```python
from build123d import *

# Parameters (mm, degrees)
F1_DEPTH = 304.8
F3_D     = 26.9875
F5_D     = 26.9875
F6_R     = 9.525


with BuildPart() as f1:
    # F0 (on Front) → F1 (new body)
    with BuildSketch(Plane.XZ):
        Polygon((12.7, 101.6), (0, 101.6), (0, 0), (101.6, 0), (101.6, 12.7), (12.7, 12.7), align=None)
    extrude(amount=F1_DEPTH)

    # F3 (through all)
    with Locations(Plane.YZ.offset(12.7)):
        with Locations((-266.7, 57.15), (-190.5, 57.15), (-114.3, 57.15), (-38.1, 57.15)):
            Hole(F3_D / 2)

    # F5 (through all)
    with Locations(Plane.XY.offset(12.7)):
        with Locations((57.15, -38.1), (57.15, -114.3), (57.15, -190.5), (57.15, -266.7)):
            Hole(F5_D / 2)

    # F6
    f6_edges = [f1.edges().sort_by_distance(p)[0] for p in [
        (12.7, -152.4, 101.6),
        (12.7, -152.4, 12.7),
        (101.6, -152.4, 12.7),
    ]]
    fillet(f6_edges, radius=F6_R)


solid = f1.part
```
For this review, take the finished solid that the model builds, in its own axes (mm). A direction names the side the tool comes from. Give positions to 0.01 mm unless a question says otherwise; leave off trailing zeros. Write each loop counter-clockwise with the first axis right and the second up, starting at its lowest first coordinate (ties: lowest second). Pieces come first, ordered by that corner, then holes. Notation, with made-up numbers: M 44,-3 L 85,-3 A26 cw 85,35 Z; hole C 40,6 d5. An arc over 180 degrees is marked long. Answer as CSV lines item,"result".
1. Draft analysis for pull direction X (two halves, no side actions). For faces 3 (the cylindrical face through (60.08, -279.87, 6.26)), 4 (the cylindrical face through (15.42, -154.53, 15.56)), 5 (the flat face through (28, -304.8, 10)), 6 (the cylindrical face through (58.91, -177.12, 6.26)), state which applies: +X half, -X half, draft (parallel to the pull), parting line (faces both ways), or undercut.
Findings:
face 3,"undercut"
face 4,"+X half"
face 5,"draft"
face 6,"undercut"
2. Consider section D-D, the plane y = -219. Write out the cut boundary in (x, z) (3 decimals).
Findings:
outline,"M 0,0 L 101.6,0 L 101.6,3.175 A9.525 ccw 92.075,12.7 L 22.225,12.7 A9.525 cw 12.7,22.225 L 12.7,92.075 A9.525 ccw 3.175,101.6 L 0,101.6 Z"
3. For faces 1 (the cylindrical face through (6.26, -279.57, 61.2)), 2 (the flat face through (58, -150, 12.7)), list the 3-axis set-ups (+Z, -Z, +X, -X, +Y, -Y) from which the entire face can be reached by the end or side of a thin tool; tool diameter is ignored.
Findings:
face 1,"+X, -X"
face 2,"+Z, +X, +Y, -Y"
4. Consider section C-C, the plane x = 57.15. Write out the cut boundary in (y, z), then the cut area to 3 significant figures.
Findings:
outline,"M -304.8,0 L -280.19,0 L -280.19,12.7 L -304.8,12.7 Z; M -253.21,0 L -203.99,0 L -203.99,12.7 L -253.21,12.7 Z; M -177.01,0 L -127.79,0 L -127.79,12.7 L -177.01,12.7 Z; M -100.81,0 L -51.59,0 L -51.59,12.7 L -100.81,12.7 Z; M -24.61,0 L 0,0 L 0,12.7 L -24.61,12.7 Z"
area,"2,500 mm2"
5. Consider section A-A, the plane z = 57.15. Write out the cut boundary in (x, y), then the cut area to 3 significant figures.
Findings:
outline,"M 0,-304.8 L 12.7,-304.8 L 12.7,-280.19 L 0,-280.19 Z; M 0,-253.21 L 12.7,-253.21 L 12.7,-203.99 L 0,-203.99 Z; M 0,-177.01 L 12.7,-177.01 L 12.7,-127.79 L 0,-127.79 Z; M 0,-100.81 L 12.7,-100.81 L 12.7,-51.59 L 0,-51.59 Z; M 0,-24.61 L 12.7,-24.61 L 12.7,0 L 0,0 Z"
area,"2,500 mm2"
6. Wall thickness on line 1 (Y direction, x = 3, z = 57); line 2 (X direction, y = -288, z = 79.5): over which ranges is each line inside the solid? List them lowest first.
Findings:
line 1,"y = -304.8 to -280.19, -253.21 to -203.99, -177.01 to -127.79, -100.81 to -51.59, -24.61 to 0"
line 2,"x = 0 to 12.7"
7. Consider section B-B, the plane y = -38.1. Write out the cut boundary in (x, z) (3 decimals).
Findings:
outline,"M 0,0 L 43.656,0 L 43.656,12.7 L 22.225,12.7 A9.525 cw 12.7,22.225 L 12.7,43.656 L 0,43.656 Z; M 0,70.644 L 12.7,70.644 L 12.7,92.075 A9.525 ccw 3.175,101.6 L 0,101.6 Z; M 70.644,0 L 101.6,0 L 101.6,3.175 A9.525 ccw 92.075,12.7 L 70.644,12.7 Z"
8. For pin 1 (5 mm diameter, centred on x = 58, y = -235.5, fed in from -Z); pin 2 (21 mm diameter, centred on y = -79, z = 67, fed in from +X); pin 3 (10 mm diameter, centred on x = 45, y = -195, fed in from +Z), all flat-tipped, find the tip position at first contact; note any pin that passes through.
Findings:
pin 1,"stops at z = 0"
pin 2,"stops at x = 12.7"
pin 3,"stops at z = 12.7"
